Here's the drawing with two shaded views (mm, measured from the low corner). I have some questions. A direction names the side the tool comes from. Round coordinates to 2 decimals unless told otherwise and drop trailing zeros. Order: outer loops, then holes, each group sorted by start corner. A loop starts at its lowest first (then second) coordinate and runs counter-clockwise, first axis right, second up.
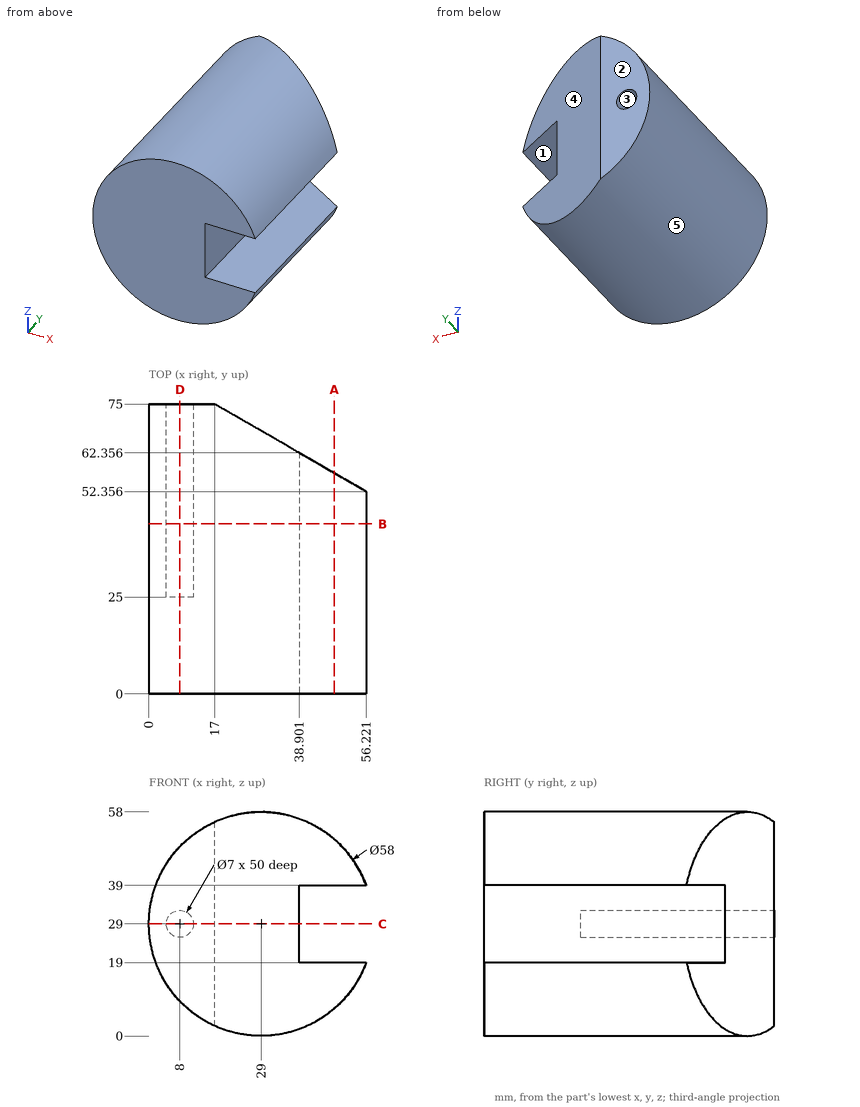
1. On a 3-axis mill with a long thin cutter (end or side, diameter ignored), from which of +Z, -Z, +X, -X, +Y, -Y can I reach the whole of each face in a straight line? I mean the marked faces 1 and 2. Say none if no direction works.
Evaluation:
face 1: +X, +Y, -Y
face 2: +Z, -Z, +X, -X, +Y
2. I'm going to push flat-ended pins straight in: P1, Ø16, axis at y = 32.5, z = 30.5, coming from the +X side; P2, Ø12, axis at x = 35.5, y = 61.5, coming from the +Z side; P3, Ø1.5, axis at x = 47.5, z = 11.5, coming from the +Y side (1 decimal). Where does each tip first touch, or does it pass through?
Evaluation:
P1: stops at x = 38.9
P2: stops at z = 58
P3: stops at y = 57.8
3. I need wall thicknesses on probe 1 along X at (y, z) = (62, 29); probe 2 along Z at (x, y) = (8, 59); probe 3 along Z at (x, y) = (39, 36.5). Which ranges of each line are inside material? Lowest first, please.
Evaluation:
probe 1: x = 0 to 4.5, 11.5 to 38.9
probe 2: z = 9 to 25.5, 32.5 to 49
probe 3: z = 1.78 to 19, 39 to 56.22
4. If we mould it in two halves opening along Z, with no side actions, what happens to the marked faces 3, 4 and 5? For each: released by +Z, released by -Z, zero draft, split by the parting line, or undercut.
Evaluation:
face 3: undercut
face 4: zero draft
face 5: split by the parting line
5. If we section it at C-C, the plane z = 29: Write out the boundary of the cut face in (x, y) (1 decimal).
Evaluation:
outline: (0, 0) - (38.9, 0) - (38.9, 62.4) - (17, 75) - (11.5, 75) - (11.5, 25) - (4.5, 25) - (4.5, 75) - (0, 75) - close
6. If we section it at B-B, the plane y = 44: Write out the boundary of the cut face in (x, z).
Evaluation:
outline: (38.9, 19) - (38.9, 39) - (56.22, 39) arc R29 ccw (long way) to (56.22, 19) - close; hole circle Ø7 at (8, 29)
7. If we section it at D-D, the plane x = 8: Write out the boundary of the cut face in (y, z), and give its area (3 significant figures).
Evaluation:
outline: (0, 9) - (75, 9) - (75, 25.5) - (25, 25.5) - (25, 32.5) - (75, 32.5) - (75, 49) - (0, 49) - close
area: 2,650 mm2
8. If we section it at A-A, the plane x = 48: Write out the boundary of the cut face in (y, z), and give its area (3 significant figures).
Evaluation:
outline: (0, 7.09) - (57.1, 7.09) - (57.1, 19) - (0, 19) - close; (0, 39) - (57.1, 39) - (57.1, 50.91) - (0, 50.91) - close
area: 1,360 mm2
